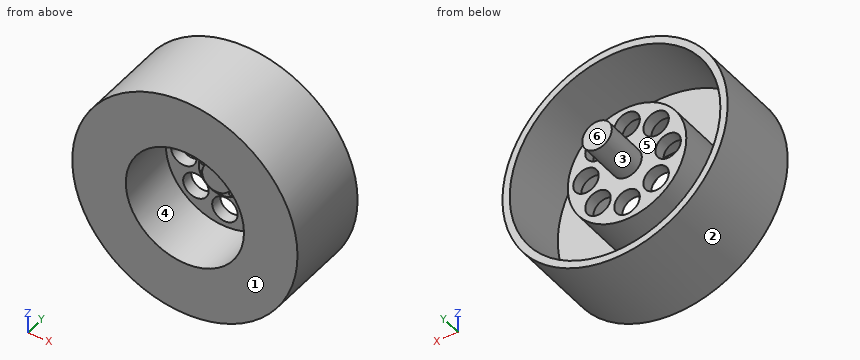
```python
from build123d import *

# Parameters (mm, degrees)
F0_R      = 19.05
F1_DEPTH  = 15
F2_R      = 10
F3_DEPTH  = 10
F4_R      = 3.75
F5_DEPTH  = 1
F6_R      = 2.5
F7_DEPTH  = 1
F8_R      = 2.1579433181
F9_DEPTH  = 18.796
F10_R     = 17.5
F10_R_2   = 2.1579433181
F11_DEPTH = 3
F13_R     = 0.385837363
F14_DEPTH = 0.2
F15_R     = 17.5
F15_R_2   = 10.0251720055
F16_DEPTH = 3
F17_R     = 17.8216148864
F17_R_2   = 10.0251720055
F18_DEPTH = 12
F12_R     = 2.5
F19_DEPTH = 7.5


with BuildPart() as f1:
    # F0 (on Front) → F1 (new body)
    with BuildSketch(Plane.XZ):
        Circle(F0_R)
    extrude(amount=F1_DEPTH)

    # F2 (on face) → F3 (cut)
    with BuildSketch(Plane.XZ.offset(15)):
        Circle(F2_R)
    extrude(amount=-F3_DEPTH, mode=Mode.SUBTRACT)

    # F4 (on face) → F5 (join)
    with BuildSketch(Plane.XZ.offset(5)):
        Circle(F4_R)
    extrude(amount=F5_DEPTH)

    # F6 (on face) → F7 (join)
    with BuildSketch(Plane.XZ.offset(6)):
        Circle(F6_R)
    extrude(amount=F7_DEPTH)

    # F8 (on face) → F9 (cut)
    with BuildSketch(Plane.XZ.offset(5)):
        with Locations((0, 6.9501847029)):
            Circle(F8_R)
        with Locations((4.9145227339, 4.9145227339)):
            Circle(F8_R)
        with Locations((6.9501847029, 0)):
            Circle(F8_R)
        with Locations((4.9145227339, -4.9145227339)):
            Circle(F8_R)
        with Locations((0, -6.9501847029)):
            Circle(F8_R)
        with Locations((-4.9145227339, -4.9145227339)):
            Circle(F8_R)
        with Locations((-6.9501847029, 0)):
            Circle(F8_R)
        with Locations((-4.9145227339, 4.9145227339)):
            Circle(F8_R)
    extrude(amount=-F9_DEPTH, mode=Mode.SUBTRACT)

    # F10 (on face) → F11 (cut)
    with BuildSketch(Plane(origin=(0, 0, 0), x_dir=(-1, 0, 0), z_dir=(0, 1, 0))):
        Circle(F10_R)
        with Locations((-4.9145227339, -4.9145227339)):
            Circle(F10_R_2, mode=Mode.SUBTRACT)
        with Locations((0, -6.9501847029)):
            Circle(F10_R_2, mode=Mode.SUBTRACT)
        with Locations((4.9145227339, -4.9145227339)):
            Circle(F10_R_2, mode=Mode.SUBTRACT)
        with Locations((-6.9501847029, 0)):
            Circle(F10_R_2, mode=Mode.SUBTRACT)
        with Locations((-4.9145227339, 4.9145227339)):
            Circle(F10_R_2, mode=Mode.SUBTRACT)
        with Locations((6.9501847029, 0)):
            Circle(F10_R_2, mode=Mode.SUBTRACT)
        with Locations((0, 6.9501847029)):
            Circle(F10_R_2, mode=Mode.SUBTRACT)
        with Locations((4.9145227339, 4.9145227339)):
            Circle(F10_R_2, mode=Mode.SUBTRACT)
    extrude(amount=-F11_DEPTH, mode=Mode.SUBTRACT)

    # F13 (on face) → F14 (join)
    with BuildSketch(Plane.XZ.offset(6)):
        with Locations((0, 3.1463524792)):
            Circle(F13_R)
        with Locations((1.8493795858, 2.545452626)):
            Circle(F13_R)
        with Locations((2.9923590279, 0.9722763864)):
            Circle(F13_R)
        with Locations((2.9923590279, -0.9722763864)):
            Circle(F13_R)
        with Locations((1.8493795858, -2.545452626)):
            Circle(F13_R)
        with Locations((0, -3.1463524792)):
            Circle(F13_R)
        with Locations((-1.8493795858, -2.545452626)):
            Circle(F13_R)
        with Locations((-2.9923590279, -0.9722763864)):
            Circle(F13_R)
        with Locations((-2.9923590279, 0.9722763864)):
            Circle(F13_R)
        with Locations((-1.8493795858, 2.545452626)):
            Circle(F13_R)
    extrude(amount=F14_DEPTH)

    # F15 (on face) → F16 (join)
    with BuildSketch(Plane(origin=(0, -3, 0), x_dir=(-1, 0, 0), z_dir=(0, 1, 0))):
        Circle(F15_R)
        Circle(F15_R_2, mode=Mode.SUBTRACT)
    extrude(amount=F16_DEPTH)

    # F17 (on face) → F18 (cut)
    with BuildSketch(Plane(origin=(0, 0, 0), x_dir=(-1, 0, 0), z_dir=(0, 1, 0))):
        Circle(F17_R)
        Circle(F17_R_2, mode=Mode.SUBTRACT)
    extrude(amount=-F18_DEPTH, mode=Mode.SUBTRACT)

    # F12 (on face) → F19 (join)
    with BuildSketch(Plane(origin=(0, -3, 0), x_dir=(-1, 0, 0), z_dir=(0, 1, 0))):
        Circle(F12_R)
    extrude(amount=F19_DEPTH)


solid = f1.part
```
Geometry: final body of the model. Coordinates: model frame, mm. Face numbers are marked on the shaded views. A direction names the side the tool comes from. Coordinates: 2 decimals unless noted, no trailing zeros. Write each loop counter-clockwise with the first axis right and the second up, starting at its lowest first coordinate (ties: lowest second). Pieces come first, ordered by that corner, then holes. Notation, with made-up numbers: M 3,2 L 19,2 A24 cw 19,30 Z; hole C 45,54.25 d8. An arc over 180 degrees is marked long. Use CSV: the item, a comma, the result in double quotes. Start each with the question number.
1. Cut plane D-D on x = 11. Return the cut outline in (y, z), plus the area to 3 significant figures.
2. First-contact query: P1, Ø1.5, axis at y = -6, z = -5, coming from the +X side; P2, Ø10, axis at x = 15, z = -6, coming from the +Y side; P3, Ø0.6, axis at x = -2, z = -2.5, coming from the -Y side; P4, Ø4, axis at y = -3, z = 2, coming from the -X side. Flat tips, straight axial feed; report the tip coordinate or a pass-through.
3. Reachability of the marked faces 4, 5 and 6 from +Z, -Z, +X, -X, +Y, -Y: full face, straight path, thin tool, end or side. Return the list, or none.
4. Cut plane A-A on y = -3.5. Count the separate pieces of the cut face and the enclosed holes in it, plus the area to 3 significant figures.
5. Ray query, probe 1 along X at (y, z) = (-4, 4); probe 2 along Y at (x, z) = (-6, 13.5); probe 3 along Z at (x, y) = (8, -4). Return the intervals inside material, ascending.
6. Mould query, pull axis Z, two halves, no side actions, for the marked faces 1, 2 and 3. Classes: pulls with the +Z half, pulls with the -Z half, needs draft (parallel to the pull), parting line crosses it, or undercut.
7. Cut plane C-C on y = -8. Return the cut outline in (x, z).
Entries:
1,outline,"M -15,-15.55 L 0,-15.55 L 0,-14.02 L -12,-14.02 L -12,14.02 L 0,14.02 L 0,15.55 L -15,15.55 Z"
1,area,"130 mm²"
2,P1,"x = 18.57"
2,P2,"y = 0"
2,P3,"y = -6.2"
2,P4,"x = -19.05"
3,face 4,"-Y"
3,face 5,"+Y"
3,face 6,"+Z, -Z, +X, -X, +Y"
4,separate pieces,"2"
4,enclosed holes,"9"
4,area,"341 mm²"
5,probe 1,"-18.63 to -17.37, -9.19 to -6.87, -2.96 to 2.96, 6.87 to 9.19, 17.37 to 18.63"
5,probe 2,"-15 to -12"
5,probe 3,"-17.29 to -15.93, -6.04 to -1.89, 1.89 to 6.04, 15.93 to 17.29"
6,face 1,"needs draft"
6,face 2,"parting line crosses it"
6,face 3,"undercut"
7,outline,"C 0,0 d38.1; C 0,0 d20.05; hole C 0,0 d35.64; hole C 0,0 d20"
